Answer from the drawing. Dimensions are ordinates in mm from the lowest x, y and z of the part. Give positions to 0.01 mm unless a question says otherwise; leave off trailing zeros. Order: outer loops, then holes, each group sorted by start corner. A loop starts at its lowest first (then second) coordinate and runs counter-clockwise, first axis right, second up. Notation, with made-up numbers: (86.25, 23.5) - (133.25, 23.5) arc R21 cw to (133.25, 56.5) - close; hole circle Ø5 at (66, 0). An arc over 180 degrees is marked (long way). Use a Markdown table: item, result. Add a question column.
1) Find section D-D, the plane x = 70. Determine the outline of the cut face in (y, z).
2) Find section B-B, the plane z = 25.4. Determine the outline of the cut face in (x, y).
3) The mould has two halves that part along Y. Classify the marked faces 1, 2 and 3: released by +Y, released by -Y, zero draft, split by the parting line, or undercut.
4) Find section A-A, the plane x = 50.8. Determine the outline of the cut face in (y, z).
5) Straight lines are drawn through the part: line 1 (X direction, y = 25, z = 3); line 2 (Z direction, x = 25.4, y = 2.25). For each, find the intervals that lie inside material, in ascending order.
6) Flat-ended cylindrical pins translate along their axes: pin 1 (12 mm diameter, centred on x = 54, y = 40.5, fed in from +Z); pin 2 (7 mm diameter, centred on x = 25.4, z = 25.4, fed in from +Y); pin 3 (5 mm diameter, centred on x = 33, y = 11, fed in from +Z); pin 4 (8 mm diameter, centred on x = 17, z = 38.5, fed in from +Y). Find the tip coordinate at first contact, or state that the pin passes through.
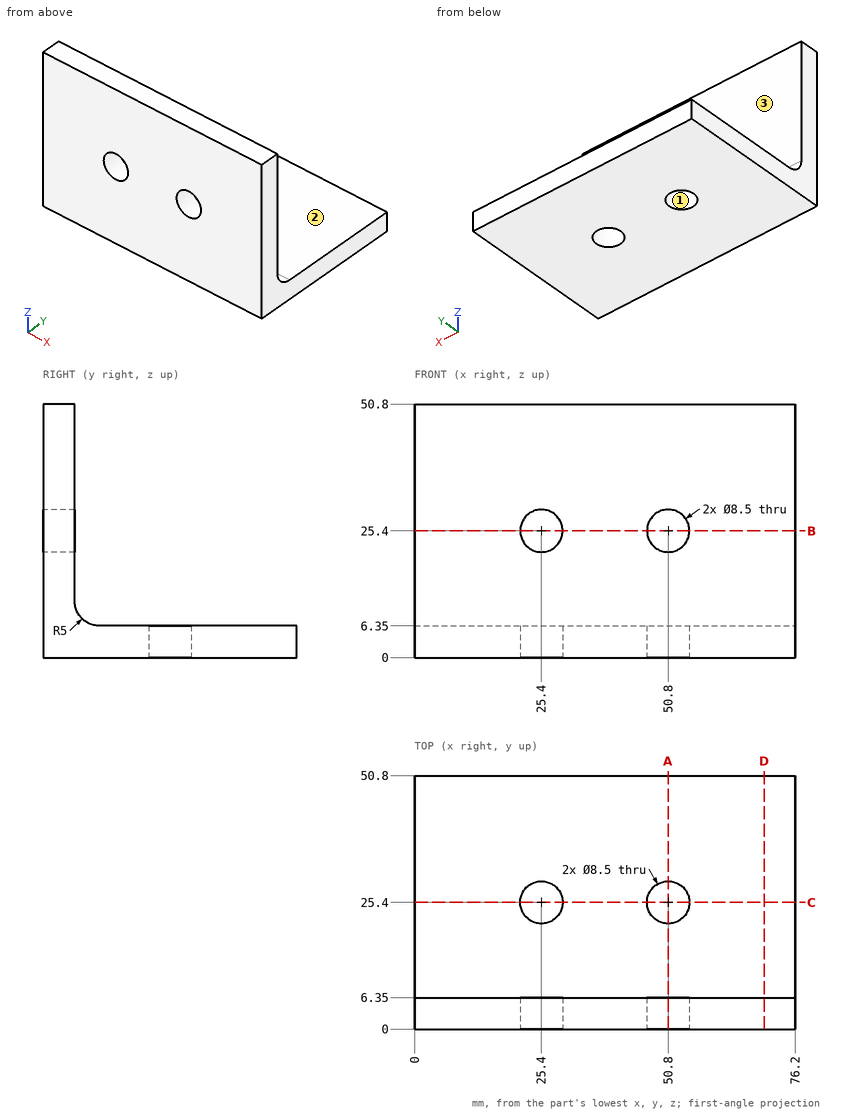
The answers:
| question | item | result |
|---|---|---|
| 1 | outline | (0, 0) - (50.8, 0) - (50.8, 6.35) - (11.35, 6.35) arc R5 cw to (6.35, 11.35) - (6.35, 50.8) - (0, 50.8) - close |
| 2 | outline | (0, 0) - (21.15, 0) - (21.15, 6.35) - (0, 6.35) - close; (29.65, 0) - (46.55, 0) - (46.55, 6.35) - (29.65, 6.35) - close; (55.05, 0) - (76.2, 0) - (76.2, 6.35) - (55.05, 6.35) - close |
| 3 | face 1 | undercut |
| 3 | face 2 | zero draft |
| 3 | face 3 | released by +Y |
| 4 | outline | (0, 0) - (21.15, 0) - (21.15, 6.35) - (11.35, 6.35) arc R5 cw to (6.35, 11.35) - (6.35, 21.15) - (0, 21.15) - close; (0, 29.65) - (6.35, 29.65) - (6.35, 50.8) - (0, 50.8) - close; (29.65, 0) - (50.8, 0) - (50.8, 6.35) - (29.65, 6.35) - close |
| 5 | line 1 | 0 to 21.17, 29.63 to 46.57, 55.03 to 76.2 |
| 5 | line 2 | 0 to 21.15, 29.65 to 50.8 |
| 6 | pin 1 | z = 6.35 |
| 6 | pin 2 | through |
| 6 | pin 3 | z = 7.24 |
| 6 | pin 4 | y = 6.35 |
